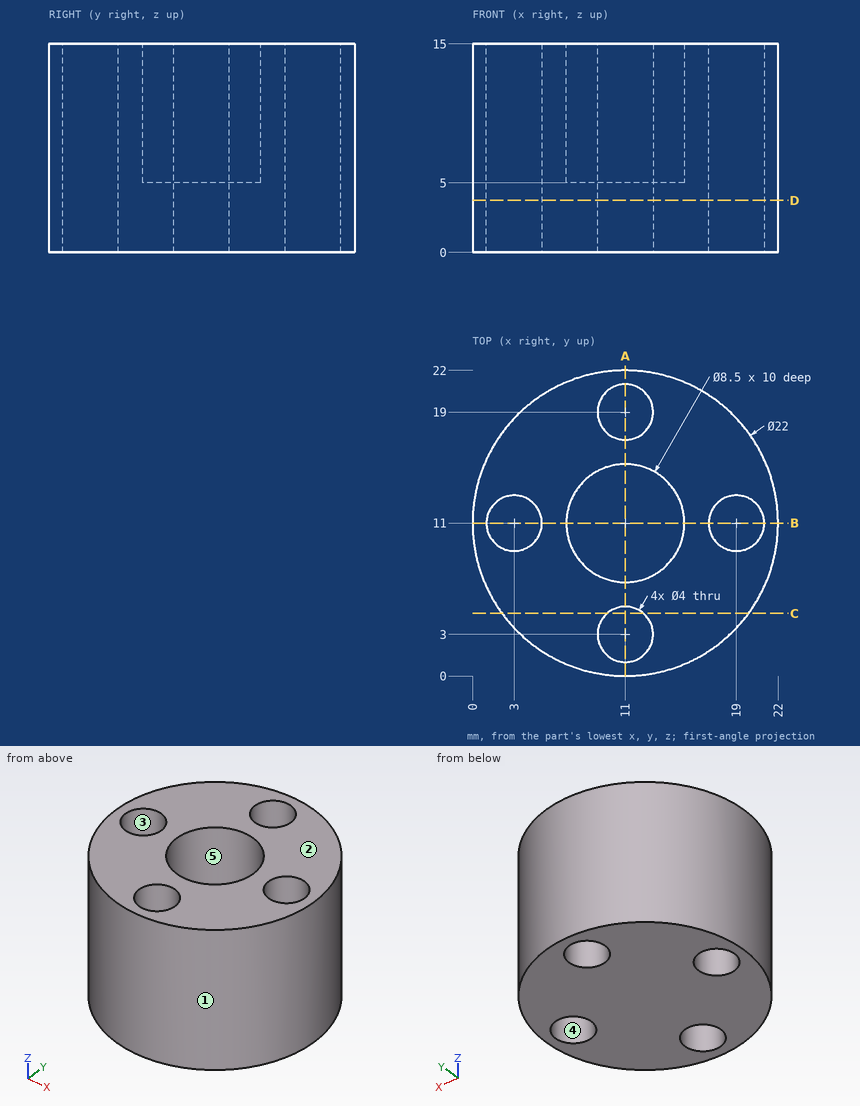
The figure shows three views and two pictorial views of one solid part (mm, origin at its lowest corner). Answer the questions. A direction names the side the tool comes from. Give positions to 0.01 mm unless a question says otherwise; leave off trailing zeros. Loops run counter-clockwise (first coordinate to the right, second up) from the corner with the lowest first, then second, coordinate; pieces in that order, holes last. Notation, with made-up numbers: (27, -15) -> (43, -15) arc R18 cw to (43, 10) -> close; hole circle Ø9 at (48, 73.25). An arc over 180 degrees is marked (long way). Put each result on its own line as item: value. Start each with the question number.
Item 1: Each of these flat-tipped pins is pushed along its axis until it touches: P1, Ø3.5, axis at x = 19, y = 11, coming from the -Z side; P2, Ø4, axis at x = 6.5, z = 5, coming from the -Y side; P3, Ø1.5, axis at x = 15.5, z = 12.5, coming from the -Y side; P4, Ø3, axis at x = 15.5, z = 3.5, coming from the +Y side. Where does it stop, or does it pass through?
Item 2: The part is cut by section D-D (z = 3.75). Give the vertices of the cut face in (x, y), then the cut area to 3 significant figures.
Item 3: The part is cut by section C-C (y = 4.5). Give the vertices of the cut face in (x, z), then the cut area to 3 significant figures.
Item 4: Which of the six approach directions +Z, -Z, +X, -X, +Y, -Y give full straight-line access (tool end or side, diameter ignored) to the marked faces 4 and 5?
Item 5: The part is cut by section A-A (x = 11). Give the vertices of the cut face in (y, z), then the cut area to 3 significant figures.
Item 6: The mould has two halves that part along Y. Classify the marked faces 1, 2 and 3: released by +Y, released by -Y, zero draft, split by the parting line, or undercut.
Item 7: Find the intervals of material crossed by L1, parallel to Y at x = 11, z = 9.25; L2, parallel to Y at x = 11, z = 3.5; L3, parallel to X at y = 10, z = 8.75, in increasing order. Write a range as [from, to].
Answers below:
1. P1: through
1. P2: y = 0.29
1. P3: y = 0.66
1. P4: y = 21.58
2. outline: circle Ø22 at (11, 11); hole circle Ø4 at (3, 11); hole circle Ø4 at (11, 3); hole circle Ø4 at (11, 19); hole circle Ø4 at (19, 11)
2. area: 330 mm2
3. outline: (2.13, 0) -> (9.68, 0) -> (9.68, 15) -> (2.13, 15) -> close; (12.32, 0) -> (19.87, 0) -> (19.87, 15) -> (12.32, 15) -> close
3. area: 227 mm2
4. face 4: +Z, -Z
4. face 5: +Z
5. outline: (0, 0) -> (1, 0) -> (1, 15) -> (0, 15) -> close; (5, 0) -> (17, 0) -> (17, 15) -> (15.25, 15) -> (15.25, 5) -> (6.75, 5) -> (6.75, 15) -> (5, 15) -> close; (21, 0) -> (22, 0) -> (22, 15) -> (21, 15) -> close
5. area: 125 mm2
6. face 1: split by the parting line
6. face 2: zero draft
6. face 3: undercut
7. L1: [0, 1], [5, 6.75], [15.25, 17], [21, 22]
7. L2: [0, 1], [5, 17], [21, 22]
7. L3: [0.05, 1.27], [4.73, 6.87], [15.13, 17.27], [20.73, 21.95]
